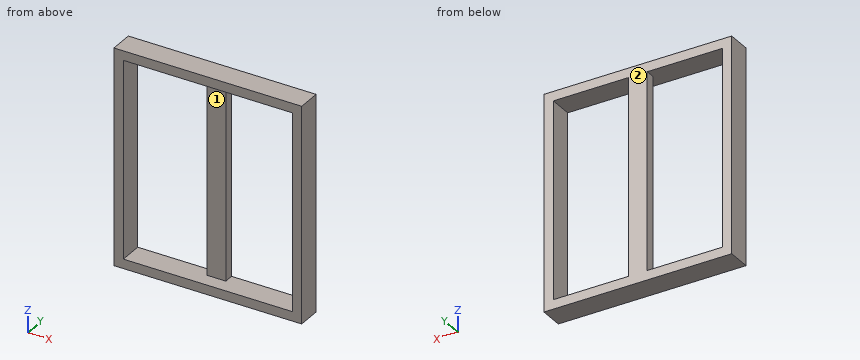
```python
from build123d import *

# Parameters (mm, degrees)
F0_W     = 20
F0_H     = 23
F1_DEPTH = 2.5
F0_W_2   = 1
F0_H_2   = 7
F0_H_3   = 6
F0_H_4   = 1
F2_DEPTH = 1


with BuildPart() as f1:
    # F0 (on Front) → F1 (new body)
    with BuildSketch(Plane.XZ):
        with Locations((-0.5926657468, -2.021088949)):
            Rectangle(F0_W, F0_H)
        Polygon((-9.5926657468, 2.478911051), (-9.5926657468, 8.478911051), (-1.5926657468, 8.478911051), (-0.5926657468, 8.478911051), (0.4073342532, 8.478911051), (8.4073342532, 8.478911051), (8.4073342532, 2.478911051), (8.4073342532, 1.478911051), (8.4073342532, -5.521088949), (8.4073342532, -6.521088949), (8.4073342532, -12.521088949), (0.4073342532, -12.521088949), (-0.5926657468, -12.521088949), (-1.5926657468, -12.521088949), (-9.5926657468, -12.521088949), (-9.5926657468, -6.521088949), (-9.5926657468, -5.521088949), (-9.5926657468, 1.478911051), align=None, mode=Mode.SUBTRACT)
    extrude(amount=F1_DEPTH)

    # F0 (on Front) → F2 (join)
    with BuildSketch(Plane.XZ):
        with Locations((-1.0926657468, -2.021088949)):
            Rectangle(F0_W_2, F0_H_2)
        with Locations((-1.0926657468, -9.521088949)):
            Rectangle(F0_W_2, F0_H_3)
        with Locations((-0.0926657468, -9.521088949)):
            Rectangle(F0_W_2, F0_H_3)
        with Locations((-1.0926657468, 5.478911051)):
            Rectangle(F0_W_2, F0_H_3)
        with Locations((-0.0926657468, 5.478911051)):
            Rectangle(F0_W_2, F0_H_3)
        with Locations((-1.0926657468, 1.978911051)):
            Rectangle(F0_W_2, F0_H_4)
        with Locations((-0.0926657468, 1.978911051)):
            Rectangle(F0_W_2, F0_H_4)
        with Locations((-0.0926657468, -2.021088949)):
            Rectangle(F0_W_2, F0_H_2)
        with Locations((-0.0926657468, -6.021088949)):
            Rectangle(F0_W_2, F0_H_4)
        with Locations((-1.0926657468, -6.021088949)):
            Rectangle(F0_W_2, F0_H_4)
    extrude(amount=F2_DEPTH)


solid = f1.part
```
Could you check a few things on this model? Use its own coordinates, in mm. Face numbers are marked on the shaded views. Round coordinates to 2 decimals unless told otherwise and drop trailing zeros. Loops run counter-clockwise (first coordinate to the right, second up) from the corner with the lowest first, then second, coordinate; pieces in that order, holes last. Notation, with made-up numbers: (-21.5, 31) - (-14.5, 31) arc R17 ccw to (-14.5, 54) - close; hole circle Ø1 at (43.5, 53). An arc over 180 degrees is marked (long way). Answer in a Markdown table with one row per item. Add a question column.
(1) I'm going to push a flat-ended pin straight in: pin 1 (0.6 mm diameter, centred on x = -0.5, z = -4, fed in from -Y). Where does the tip first touch, or does it pass through?
(2) If we section it at C-C (z = 5.75): Please give me the cut outline in (x, y), plus the area to 3 significant figures.
(3) If we section it at D-D (x = 0): Please give me the cut outline in (y, z), plus the area to 3 significant figures.
(4) If we mould it in two halves opening along X, with no side actions, what happens to the marked faces 1 and 2? For each: pulls with the +X half, pulls with the -X half, needs draft (parallel to the pull), parting line crosses it, or undercut.
(5) If we section it at B-B (y = -0.65): Please give me the cut outline in (x, z), plus the area to 3 significant figures.
(6) I need wall thicknesses on line 1 along X through (y, z) = (-0.85, 3.25); line 2 along Z through (x, y) = (5.5, -0.6); line 3 along X through (y, z) = (-1.65, 4). Which ranges of each line are inside material? Lowest first, please.
(7) If we section it at A-A (x = 6): Please give me the cut outline in (y, z).
Model answer:
| question | item | result |
|---|---|---|
| 1 | pin 1 | stops at y = -1 |
| 2 | outline | (-10.59, -2.5) - (-9.59, -2.5) - (-9.59, 0) - (-10.59, 0) - close; (-1.59, -1) - (0.41, -1) - (0.41, 0) - (-1.59, 0) - close; (8.41, -2.5) - (9.41, -2.5) - (9.41, 0) - (8.41, 0) - close |
| 2 | area | 7.00 mm² |
| 3 | outline | (-2.5, -13.52) - (0, -13.52) - (0, 9.48) - (-2.5, 9.48) - (-2.5, 8.48) - (-1, 8.48) - (-1, -12.52) - (-2.5, -12.52) - close |
| 3 | area | 26.0 mm² |
| 4 | face 1 | undercut |
| 4 | face 2 | needs draft |
| 5 | outline | (-10.59, -13.52) - (9.41, -13.52) - (9.41, 9.48) - (-10.59, 9.48) - close; hole (-9.59, -12.52) - (-1.59, -12.52) - (-1.59, 8.48) - (-9.59, 8.48) - close; hole (0.41, -12.52) - (8.41, -12.52) - (8.41, 8.48) - (0.41, 8.48) - close |
| 5 | area | 124 mm² |
| 6 | line 1 | x = -10.59 to -9.59, -1.59 to 0.41, 8.41 to 9.41 |
| 6 | line 2 | z = -13.52 to -12.52, 8.48 to 9.48 |
| 6 | line 3 | x = -10.59 to -9.59, 8.41 to 9.41 |
| 7 | outline | (-2.5, -13.52) - (0, -13.52) - (0, -12.52) - (-2.5, -12.52) - close; (-2.5, 8.48) - (0, 8.48) - (0, 9.48) - (-2.5, 9.48) - close |
